Source: CAD feature listing. Evaluate the final solid. Frame: model axes, mm. Face numbers are marked on the shaded views. A direction names the side the tool comes from. Give positions to 0.01 mm unless a question says otherwise; leave off trailing zeros. Write each loop counter-clockwise with the first axis right and the second up, starting at its lowest first coordinate (ties: lowest second). Pieces come first, ordered by that corner, then holes. Notation, with made-up numbers: M 89.25,72.25 L 141.25,72.25 A6 ccw 141.25,76.25 Z; hole C 80.5,33.25 d2. An arc over 180 degrees is marked long. Return JSON: item names as keys, results as strings.
Autodesk Inventor part; units mm, degrees
ref_plane "YZ Plane" through (0, 0, 0) normal (1, 0, 0) x (0, 1, 0)
ref_plane "XZ Plane" through (0, 0, 0) normal (0, 1, 0) x (-1, 0, 0)
ref_plane "XY Plane" through (0, 0, 0) normal (0, 0, 1) x (1, 0, 0)
sketch "Sketch1" plane through (0, 0, 0) normal (0, 0, 1) x (1, 0, 0)
  line L0 (-25.7967, 11.5978) -> (431.4033, 11.5978)
  line L1 (431.4033, 11.5978) -> (431.4033, -293.2022)
  line L2 (431.4033, -293.2022) -> (-25.7967, -293.2022)
  line L3 (-25.7967, -293.2022) -> (-25.7967, 11.5978)
  point P0 (0, 0)
  dimension "d0" = 457.2
  dimension "d1" = 304.8
extrude "Extrusion1" add sketch "Sketch1" along normal blind 457.2
sketch "Sketch2" plane through (-25.7967, 11.5978, 0) normal (0, 1, 0) x (1, 0, 0)
  line L0 (0, 0) -> (0, -457.2)
  line L1 (0, -457.2) -> (0, -452.2)
  line L2 (0, -457.2) -> (457.2, -457.2)
  line L3 (0, -457.2) -> (5, -457.2)
  line L4 (5, -452.2) -> (452, -452.2)
  line L5 (452, -452.2) -> (452, -5.2)
  line L6 (452, -5.2) -> (5, -5.2)
  line L7 (452, -5.2) -> (899, -5.2) construction
  line L8 (5, -452.2) -> (5, -5.2)
  point P0 (25.7967, 0)
  dimension "d4" = 5
  dimension "d5" = 5
  dimension "d6" = 447
  dimension "d7" = 447
  dimension "d8" = 447
  dimension "d9" = 180
extrude "Extrusion2" cut sketch "Sketch2" against normal blind 294
sketch "Sketch3" plane through (426.2033, 11.5978, 452.2) normal (0, 0, -1) x (-1, 0, 0)
  point P0 (426.2033, -11.5978)
properties part number "rectangle box" material "Glass"
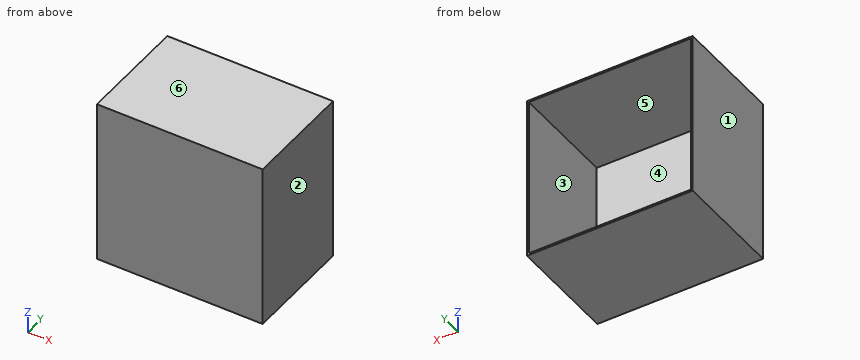
1) Cut plane B-B, the plane z = 340.5. Return the cut outline in (x, y).
Numbers:
{"outline": "M -25.8,-293.2 L 431.4,-293.2 L 431.4,11.6 L 426.2,11.6 L 426.2,-282.4 L -20.8,-282.4 L -20.8,11.6 L -25.8,11.6 Z"}
2) Cut plane A-A, the plane y = -26.5. Return the cut outline in (x, z).
Numbers:
{"outline": "M -25.8,0 L 431.4,0 L 431.4,457.2 L -25.8,457.2 Z; hole M -20.8,5.2 L 426.2,5.2 L 426.2,452.2 L -20.8,452.2 Z"}
3) Cut plane C-C, the plane x = 195.5. Return the cut outline in (y, z).
Numbers:
{"outline": "M -293.2,0 L 11.6,0 L 11.6,5.2 L -282.4,5.2 L -282.4,452.2 L 11.6,452.2 L 11.6,457.2 L -293.2,457.2 Z"}
4) Draft query along X for the marked faces 1, 2, 3 and 4. Return one class per face: released by +X, released by -X, zero draft, split by the parting line, or undercut.
Numbers:
{"face 1": "released by -X", "face 2": "released by +X", "face 3": "undercut", "face 4": "undercut"}
5) Contact query for a flat-ended pin moving along its axis: pin 1 Ø5 at (x, z) = (297.5, 132.5) entering from +Y. Output: stop coordinate, or through.
Numbers:
{"pin 1": "stops at y = -282.4"}
6) Line query: line 1 (Z direction, x = 54, y = -263.5); line 2 (X direction, y = -127.5, z = 200.5); line 3 (Y direction, x = 89, z = 245). Output: solid intervals per line, ascending. Write a range as [from, to].
Numbers:
{"line 1": "z = [0, 5.2], [452.2, 457.2]", "line 2": "x = [-25.8, -20.8], [426.2, 431.4]", "line 3": "y = [-293.2, -282.4]"}
7) Set-up query: the marked faces 5 and 6. Return all of +Z, -Z, +X, -X, +Y, -Y with unobstructed straight access to the full face (end or side cutting, diameter ignored); none if empty.
Numbers:
{"face 5": "+Y", "face 6": "+Z, +X, -X, +Y, -Y"}
